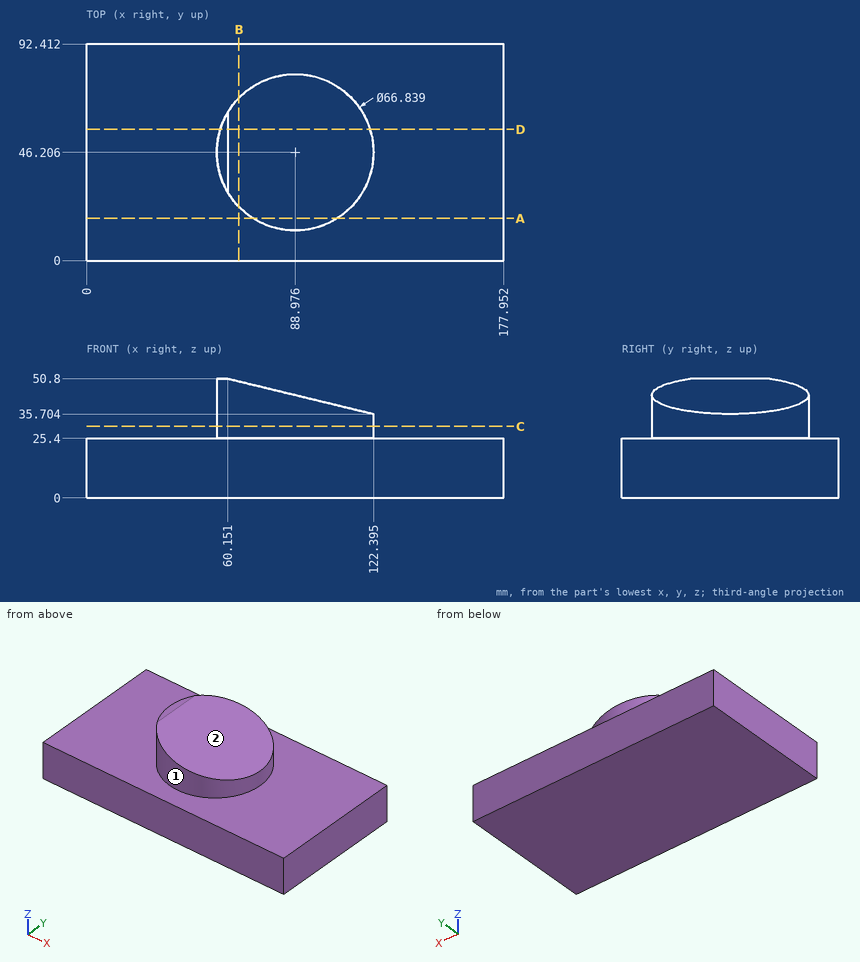
The drawing under review shows one solid part. Ordinate dimensions are in mm from its lowest x, y, z. A direction names the side the tool comes from. Give positions to 0.01 mm unless a question says otherwise; leave off trailing zeros. Order: outer loops, then holes, each group sorted by start corner. A loop starts at its lowest first (then second) coordinate and runs counter-clockwise, first axis right, second up. Notation, with made-up numbers: M 47,74.25 L 81,74.25 A25 ccw 81,92.25 Z; hole C 81,-5 d7. An arc over 180 degrees is marked long. Answer in a Markdown table with one row per item. Add a question column.
1. Add section B-B on x = 65. State the section outline as (y, z) points (1 decimal).
2. Machinability: for the marked faces 1 and 2, which of the approach directions +Z, -Z, +X, -X, +Y, -Y give a long, thin tool a straight path to every point of the face, cutting with its end or side? Answer none if there is none.
3. Add section A-A on y = 18. State the section outline as (x, z) points, plus the area to 3 significant figures.
4. To check wall thickness, follow line 1 along Z through (x, y) = (66, 14.5); line 2 along Z through (x, y) = (77.5, 49); line 3 along Y through (x, z) = (63.5, 28) (1 decimal). State the ranges of each line that lie inside material, in increasing order.
5. Add section D-D on y = 56. State the section outline as (x, z) points.
6. For pin 1 Ø1.5 at (x, y) = (22, 76.5) entering from +Z; pin 2 Ø10 at (x, z) = (65.5, 35) entering from +Y (1 decimal); pin 3 Ø10 at (x, y) = (33.5, 25) entering from -Z; pin 4 Ø12 at (x, z) = (115.5, 35) entering from +Y, all flat-tipped, find the tip position at first contact; note any pin that passes through.
7. Add section C-C on z = 30.5. State the section outline as (x, y) points (1 decimal), plus the area to 3 significant figures.
The answers:
| question | item | result |
|---|---|---|
| 1 | outline | M 0,0 L 92.4,0 L 92.4,25.4 L 69.5,25.4 L 69.5,49.6 L 22.9,49.6 L 22.9,25.4 L 0,25.4 Z |
| 2 | face 1 | +Z |
| 2 | face 2 | +Z, +X, +Y, -Y |
| 3 | outline | M 0,0 L 177.95,0 L 177.95,25.4 L 106.9,25.4 L 106.9,39.46 L 71.05,48.16 L 71.05,25.4 L 0,25.4 Z |
| 3 | area | 5,180 mm2 |
| 4 | line 1 | 0 to 25.4 |
| 4 | line 2 | 0 to 46.59 |
| 4 | line 3 | 24.6 to 67.8 |
| 5 | outline | M 0,0 L 177.95,0 L 177.95,25.4 L 120.93,25.4 L 120.93,36.06 L 60.15,50.8 L 57.02,50.8 L 57.02,25.4 L 0,25.4 Z |
| 6 | pin 1 | z = 25.4 |
| 6 | pin 2 | y = 74.1 |
| 6 | pin 3 | z = 0 |
| 6 | pin 4 | y = 72.58 |
| 7 | outline | C 89,46.2 d66.8 |
| 7 | area | 3,510 mm2 |
